Study the drawing (mm; zero at the part's minimum x, y, z) and answer. Coordinates: 2 decimals unless noted, no trailing zeros. Order: outer loops, then holes, each group sorted by start corner. A loop starts at its lowest first (then second) coordinate and runs counter-clockwise, first axis right, second up.
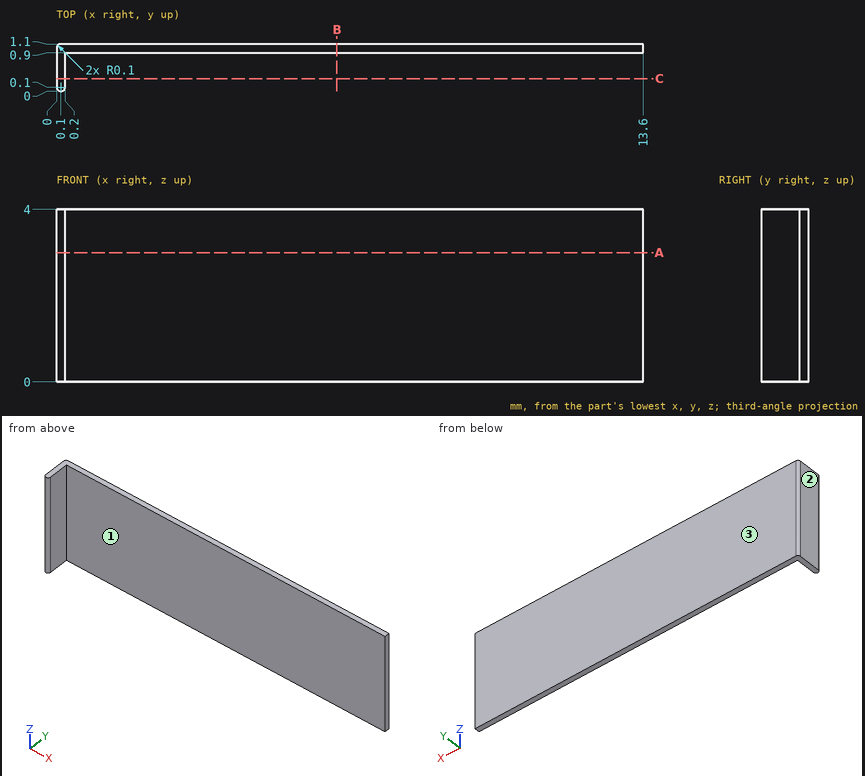
1) Straight lines are drawn through the part: line 1 (X direction, y = 0.55, z = 1.9); line 2 (Y direction, x = 5.5, z = 1.9). For each, find the intervals that lie inside material, in ascending order.
A:
line 1: x = 0 to 0.2
line 2: y = 0.9 to 1.1
2) A cutting plane is placed at C-C, the plane y = 0.3. Determine the outline of the cut face in (x, z), and give its area (3 significant figures).
A:
outline: (0, 0) - (0.2, 0) - (0.2, 4) - (0, 4) - close
area: 0.800 mm2
3) Flat-ended cylindrical pins translate along their axes: pin 1 Ø1.5 at (x, z) = (7.5, 2) entering from -Y; pin 2 Ø0.6 at (y, z) = (0.5, 1.5) entering from +X. Find the tip coordinate at first contact, or state that the pin passes through.
A:
pin 1: stops at y = 0.9
pin 2: stops at x = 0.2
4) Determine the mould class of the marked faces 1, 2 and 3 for opening direction Y: pulls with the +Y half, pulls with the -Y half, needs draft (parallel to the pull), parting line crosses it, or undercut.
A:
face 1: pulls with the -Y half
face 2: needs draft
face 3: pulls with the +Y half
5) A cutting plane is placed at A-A, the plane z = 3. Determine the outline of the cut face in (x, y).
A:
outline: (0, 0.1) arc R0.1 ccw to (0.2, 0.1) - (0.2, 0.9) - (13.6, 0.9) - (13.6, 1.1) - (0.1, 1.1) arc R0.1 ccw to (0, 1) - close
6) A cutting plane is placed at B-B, the plane x = 6.5. Determine the outline of the cut face in (y, z).
A:
outline: (0.9, 0) - (1.1, 0) - (1.1, 4) - (0.9, 4) - close
